```python
from build123d import *

# Parameters (mm, degrees)
F1_DEPTH = 3.175


# Not quite as in the source:
# - ends of sketch curves that miss each other by under 0.0002 mm in the source are joined


with BuildPart() as f1:
    # F0 (on Right) → F1 (new body)
    with BuildSketch(Plane.YZ):
        with BuildLine():
            ThreePointArc((95.7616986955, -2.4384445977), (115.8206686741, 16.458433146), (138.7853580017, 31.6925169435))
            ThreePointArc((138.7853580017, 31.6925169435), (140.2492541442, 34.5947643313), (138.0609974389, 36.9984236581))
            ThreePointArc((138.0609974389, 36.9984236581), (-3.331363766, 42.4083585784), (-136.5310363288, -5.3296204889))
            ThreePointArc((-136.5310363288, -5.3296204889), (-140.275599037, -12.4275830619), (-136.5310425411, -19.5255553241))
            ThreePointArc((-136.5310425411, -19.5255553241), (-85.3689517348, -37.3376085714), (-31.987598638, -46.5712291765))
            ThreePointArc((-31.987598638, -46.5712291765), (-6.7583016255, -41.5949042645), (11.8270849627, -23.8223232356))
            Line((11.8270849627, -23.8223232356), (12.4481411913, -22.7466161766))
            ThreePointArc((12.4481411913, -22.7466161766), (19.971713381, -14.8813600309), (30.2742956681, -11.3709138521))
            Line((30.2742956681, -11.3709138521), (88.2365367651, -6.2104608931))
            ThreePointArc((88.2365367651, -6.2104608931), (92.3577760693, -5.0399785829), (95.7616986955, -2.4384445977))
        make_face()
    extrude(amount=F1_DEPTH)


solid = f1.part
```
Check sheet for the modelled part. Datum: model origin and axes. Units: mm. Give positions to 0.01 mm unless a question says otherwise; leave off trailing zeros. Order: outer loops, then holes, each group sorted by start corner. A loop starts at its lowest first (then second) coordinate and runs counter-clockwise, first axis right, second up. Notation, with made-up numbers: M -34.5,23.25 L 22.5,23.25 A36 ccw 22.5,59.25 Z; hole C 37.5,-31 d11. An arc over 180 degrees is marked long. Answer in a Markdown table with one row per item.
1) Thickness scan on L1, parallel to Z at x = 1, y = 15; L2, parallel to Y at x = 1.45, z = 3.5; L3, parallel to Z at x = 2, y = 35. Record the ranges inside material, lowest first. Write a range as [from, to].
Filled sheet:
| item | result |
|---|---|
| L1 | z = [-19.17, 44.77] |
| L2 | y = [-120.79, 101.35] |
| L3 | z = [-10.95, 46.3] |
2) Cross-section at C-C, the plane z = -31. Enter the section's corners in (x, y) (3 decimals), plus the area to 3 significant figures.
Filled sheet:
| item | result |
|---|---|
| outline | M 0,-106.845 L 3.175,-106.845 L 3.175,6.704 L 0,6.704 Z |
| area | 361 mm2 |
3) Gauge pin test, flat end, axial feed: P1, Ø1.5, axis at x = 3, z = 0, coming from the -Y side. Record the tip position at first contact, or that the pin passes through.
Filled sheet:
| item | result |
|---|---|
| P1 | stops at y = -128.59 |
4) Cross-section at A-A, the plane x = 2.1. Enter the section's corners in (y, z).
Filled sheet:
| item | result |
|---|---|
| outline | M -136.53,-19.53 A331.21 ccw -31.99,-46.57 A45.86 ccw 11.83,-23.82 L 12.45,-22.75 A22.93 cw 30.27,-11.37 L 88.24,-6.21 A11.47 ccw 95.76,-2.44 A162.44 cw 138.79,31.69 A2.87 ccw 138.06,37 A372.31 ccw -136.53,-5.33 A8.6 ccw Z |
5) Cross-section at B-B, the plane y = -107. Enter the section's corners in (x, z) (3 decimals), plus the area to 3 significant figures.
Filled sheet:
| item | result |
|---|---|
| outline | M 0,-30.948 L 3.175,-30.948 L 3.175,10.435 L 0,10.435 Z |
| area | 131 mm2 |
